from build123d import *

# Parameters (mm, degrees)
F0_R     = 50.796035682
F1_DEPTH = 6.35
F0_R_2   = 25.5997355282
F2_DEPTH = 6.35


with BuildPart() as f1:
    # F0 (on Top) → F1 (new body)
    with BuildSketch(Plane.XY):
        Circle(F0_R)
        with BuildLine():
            ThreePointArc((39.3271974597, 7.2596428653), (39.8251792413, 3.6449928619), (39.9916350574, 0))
            ThreePointArc((39.9916350574, 0), (37.8457361774, -12.9240522963), (31.638331797, -24.4611290759))
            ThreePointArc((31.638331797, -24.4611290759), (32.6975616463, -25.8682109338), (33.0734716269, -27.5888325992))
            ThreePointArc((33.0734716269, -27.5888325992), (30.4751171589, -31.421463006), (25.9528595707, -30.4266323255))
            ThreePointArc((25.9528595707, -30.4266323255), (11.2745427029, -38.3694613124), (-5.3673629967, -39.6298156572))
            ThreePointArc((-5.3673629967, -39.6298156572), (-10.3899431598, -42.8710411012), (-13.3713628706, -37.6900189645))
            ThreePointArc((-13.3713628706, -37.6900189645), (-27.5888779577, -28.9514194402), (-37.0021800615, -15.1713396))
            ThreePointArc((-37.0021800615, -15.1713396), (-42.3272537393, -12.438997445), (-39.3271186708, -7.2600696702))
            ThreePointArc((-39.3271186708, -7.2600696702), (-38.8660161768, 9.4214468691), (-31.637317072, 24.4624414777))
            ThreePointArc((-31.637317072, 24.4624414777), (-31.9331144569, 30.4341189249), (-25.9541217074, 30.4255557215))
            ThreePointArc((-25.9541217074, 30.4255557215), (-11.2785991848, 38.3682691165), (5.3606272578, 39.6307273459))
            ThreePointArc((5.3606272578, 39.6307273459), (9.8039037737, 42.9758363595), (13.548769251, 38.8638486327))
            ThreePointArc((13.548769251, 38.8638486327), (13.5057955215, 38.2696140057), (13.3777686423, 37.6877457633))
            ThreePointArc((13.3777686423, 37.6877457633), (27.5911811268, 28.9492244903), (37.0020154097, 15.1717411718))
            ThreePointArc((37.0020154097, 15.1717411718), (40.7552771421, 14.6424823027), (42.495179297, 11.2750160335))
            ThreePointArc((42.495179297, 11.2750160335), (41.6078280146, 8.7177063827), (39.3271974597, 7.2596428653))
        make_face(mode=Mode.SUBTRACT)
    extrude(amount=F1_DEPTH)



with BuildPart() as f1b:
    # F0 (on Top) → F1, piece 2 (new body)
    with BuildSketch(Plane.XY):
        with BuildLine():
            Line((29.9194537324, -23.5791233665), (37.3940186124, 7.2624677043))
            ThreePointArc((37.3940186124, 7.2624677043), (34.4052772179, 10.1109124169), (35.3777320032, 14.1234607462))
            Line((35.3777320032, 14.1234607462), (12.4084521668, 36.0145229256))
            ThreePointArc((12.4084521668, 36.0145229256), (8.4460308303, 34.8500592639), (5.4563650491, 37.6993849709))
            Line((5.4563650491, 37.6993849709), (-24.9908830503, 28.7516454448))
            ThreePointArc((-24.9908830503, 28.7516454448), (-24.8656043881, 28.1762274896), (-24.8235590671, 27.5888325992))
            ThreePointArc((-24.8235590671, 27.5888325992), (-26.3979468028, 24.3473427918), (-29.9190635285, 23.5807334278))
            Line((-29.9190635285, 23.5807334278), (-37.3941206986, -7.2628889331))
            ThreePointArc((-37.3941206986, -7.2628889331), (-35.1217260633, -8.7227134695), (-34.2382009209, -11.2750160335))
            ThreePointArc((-34.2382009209, -11.2750160335), (-34.5337408719, -12.8088983718), (-35.3780457549, -14.1231617225))
            Line((-35.3780457549, -14.1231617225), (-12.4035384742, -36.019205961))
            ThreePointArc((-12.4035384742, -36.019205961), (-8.4476296116, -34.8566561642), (-5.4628775231, -37.7012988359))
            Line((-5.4628775231, -37.7012988359), (24.9892935944, -28.752112549))
            ThreePointArc((24.9892935944, -28.752112549), (25.9610603149, -24.7424033164), (29.9194537324, -23.5791233665))
        make_face()
        Circle(F0_R_2, mode=Mode.SUBTRACT)
    extrude(amount=F1_DEPTH)


with BuildPart() as f1_1:
    add(f1.part)

    add(f1b.part)  # F2 merges F1b
    # F0 (on Top) → F2 (join)
    with BuildSketch(Plane.XY):
        with BuildLine():
            ThreePointArc((31.638331797, -24.4611290759), (37.8457361774, -12.9240522963), (39.9916350574, 0))
            ThreePointArc((39.9916350574, 0), (39.8251792413, 3.6449928619), (39.3271974597, 7.2596428653))
            ThreePointArc((39.3271974597, 7.2596428653), (38.3604403722, 7.146314542), (37.3940186124, 7.2624677043))
            Line((37.3940186124, 7.2624677043), (29.9194537324, -23.5791233665))
            ThreePointArc((29.9194537324, -23.5791233665), (30.8312469464, -23.9180968879), (31.638331797, -24.4611290759))
        make_face()
        with BuildLine():
            ThreePointArc((35.3777320032, 14.1234607462), (36.1276546961, 14.7440077063), (37.0020154097, 15.1717411718))
            ThreePointArc((37.0020154097, 15.1717411718), (27.5911811268, 28.9492244903), (13.3777686423, 37.6877457633))
            ThreePointArc((13.3777686423, 37.6877457633), (12.9924184393, 36.7936041028), (12.4084521668, 36.0145229256))
            Line((12.4084521668, 36.0145229256), (35.3777320032, 14.1234607462))
        make_face()
        with BuildLine():
            ThreePointArc((-5.3673629967, -39.6298156572), (11.2745427029, -38.3694613124), (25.9528595707, -30.4266323255))
            ThreePointArc((25.9528595707, -30.4266323255), (25.3716802728, -29.6465678813), (24.9892935944, -28.752112549))
            Line((24.9892935944, -28.752112549), (-5.4628775231, -37.7012988359))
            ThreePointArc((-5.4628775231, -37.7012988359), (-5.3376272012, -38.2765866213), (-5.2955913916, -38.8638486327))
            ThreePointArc((-5.2955913916, -38.8638486327), (-5.3135735047, -39.2485097322), (-5.3673629967, -39.6298156572))
        make_face()
        with BuildLine():
            ThreePointArc((5.4563650491, 37.6993849709), (5.2938683757, 38.6593739913), (5.3606272578, 39.6307273459))
            ThreePointArc((5.3606272578, 39.6307273459), (-11.2785991848, 38.3682691165), (-25.9541217074, 30.4255557215))
            ThreePointArc((-25.9541217074, 30.4255557215), (-25.3731377903, 29.6457791632), (-24.9908830503, 28.7516454448))
            Line((-24.9908830503, 28.7516454448), (5.4563650491, 37.6993849709))
        make_face()
        with BuildLine():
            ThreePointArc((-37.0021800615, -15.1713396), (-27.5888779577, -28.9514194402), (-13.3713628706, -37.6900189645))
            ThreePointArc((-13.3713628706, -37.6900189645), (-12.9866339101, -36.7971602183), (-12.4035384742, -36.019205961))
            Line((-12.4035384742, -36.019205961), (-35.3780457549, -14.1231617225))
            ThreePointArc((-35.3780457549, -14.1231617225), (-36.1278992542, -14.7436496905), (-37.0021800615, -15.1713396))
        make_face()
        with BuildLine():
            ThreePointArc((-29.9190635285, 23.5807334278), (-30.8305291615, 23.9195906141), (-31.637317072, 24.4624414777))
            ThreePointArc((-31.637317072, 24.4624414777), (-38.8660161768, 9.4214468691), (-39.3271186708, -7.2600696702))
            ThreePointArc((-39.3271186708, -7.2600696702), (-38.3604523499, -7.1467479477), (-37.3941206986, -7.2628889331))
            Line((-37.3941206986, -7.2628889331), (-29.9190635285, 23.5807334278))
        make_face()
    extrude(amount=F2_DEPTH)


solid = f1_1.part
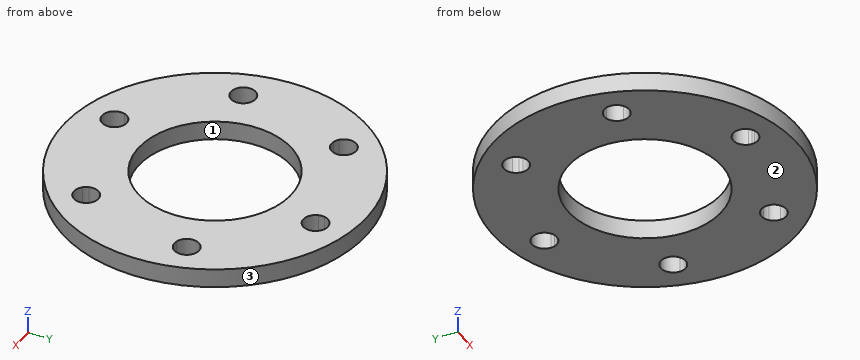
Model file for the job. Use its own axes, mm. Face numbers are marked on the shaded views. Coordinates: 2 decimals unless noted, no trailing zeros. Write each loop counter-clockwise with the first axis right and the second up, starting at its lowest first coordinate (ties: lowest second). Pieces come first, ordered by that corner, then holes. Notation, with made-up numbers: (-19, -38) -> (19, -38) arc R18 cw to (19, -16) -> close; hole circle Ø2 at (38, 72.5). An arc over 180 degrees is marked (long way). One line per item, written item: value. Start each with the question number.
1) Pull direction X, two halves, no side cores. Call the marked faces 1, 2 and 3: +X half, -X half, draft (parallel to the pull), parting line (faces both ways), or undercut.
2) Slice it at A-A on x = 0. Write the cut outline in (y, z).
3) Probe probe 1 along Y at (x, z) = (0, 4.5); probe 2 along X at (y, z) = (-8.5, 3.25); probe 3 along X at (y, z) = (-11.5, 6). List the from-to ranges inside material, lowest first.
4) Slice it at C-C on z = 4.25. Write the cut outline in (x, y).
5) Flat gauge pins, fed straight in: pin 1 Ø3 at (x, z) = (6.5, 2.5) entering from -Y; pin 2 Ø1 at (y, z) = (-29.5, 4) entering from -X; pin 3 Ø2 at (x, z) = (26, 4) entering from -Y. Where does each tip first touch, or does it go through?
Answers follow:
1. face 1: undercut
1. face 2: draft
1. face 3: parting line
2. outline: (-50.8, 0) -> (-25.6, 0) -> (-25.6, 6.35) -> (-50.8, 6.35) -> close; (25.6, 0) -> (50.8, 0) -> (50.8, 6.35) -> (25.6, 6.35) -> close
3. probe 1: -50.8 to -25.6, 25.6 to 50.8
3. probe 2: -50.08 to -41.42, -35.31 to -24.15, 24.15 to 50.08
3. probe 3: -49.48 to -42.49, -34.24 to -22.87, 22.87 to 49.48
4. outline: circle Ø101.59 at (0, 0); hole circle Ø8.26 at (-38.37, -11.28); hole circle Ø8.25 at (-28.95, 27.59); hole circle Ø51.2 at (0, 0); hole circle Ø8.25 at (-9.42, -38.86); hole circle Ø8.26 at (9.42, 38.86); hole circle Ø8.25 at (28.95, -27.59); hole circle Ø8.26 at (38.37, 11.28)
5. pin 1: y = -50.55
5. pin 2: x = -41.7
5. pin 3: y = -44.22
